from build123d import *

# Parameters (mm, degrees)
SKETCH1_W           = 100
SKETCH1_H           = 120
SKETCH1_R           = 2.6
SKETCH1_R_2         = 3.55
BOSS_EXTRUDE1_DEPTH = 3.2
FILLET1_R           = 10


with BuildPart() as part:
    # Sketch1 → Boss-Extrude1 (new body)
    with BuildSketch(Plane.XY):
        Rectangle(SKETCH1_W, SKETCH1_H)
        Circle(SKETCH1_R, mode=Mode.SUBTRACT)
        with Locations((0, 10)):
            Circle(SKETCH1_R, mode=Mode.SUBTRACT)
        with Locations((0, 42.3)):
            Circle(SKETCH1_R, mode=Mode.SUBTRACT)
        with Locations((0, -10)):
            Circle(SKETCH1_R, mode=Mode.SUBTRACT)
        with Locations((10, -20)):
            Circle(SKETCH1_R, mode=Mode.SUBTRACT)
        with Locations((10, 0)):
            Circle(SKETCH1_R, mode=Mode.SUBTRACT)
        with Locations((-10, 0)):
            Circle(SKETCH1_R, mode=Mode.SUBTRACT)
        with Locations((-32.3, 0)):
            Circle(SKETCH1_R_2, mode=Mode.SUBTRACT)
        with Locations((35.25, 0)):
            Circle(SKETCH1_R, mode=Mode.SUBTRACT)
        with Locations((35.25, 42.3)):
            Circle(SKETCH1_R, mode=Mode.SUBTRACT)
        with Locations((10, -30)):
            Circle(SKETCH1_R, mode=Mode.SUBTRACT)
        with Locations((-10, -20)):
            Circle(SKETCH1_R, mode=Mode.SUBTRACT)
        with Locations((-32.3, 42.3)):
            Circle(SKETCH1_R_2, mode=Mode.SUBTRACT)
        with Locations((-22.3, 42.3)):
            Circle(SKETCH1_R_2, mode=Mode.SUBTRACT)
        with Locations((-10, -30)):
            Circle(SKETCH1_R, mode=Mode.SUBTRACT)
        with Locations((-40, 10)):
            Circle(SKETCH1_R, mode=Mode.SUBTRACT)
        with Locations((-20, 10)):
            Circle(SKETCH1_R, mode=Mode.SUBTRACT)
        with Locations((20, 10)):
            Circle(SKETCH1_R, mode=Mode.SUBTRACT)
        with Locations((40, 10)):
            Circle(SKETCH1_R, mode=Mode.SUBTRACT)
        with Locations((40, -10)):
            Circle(SKETCH1_R, mode=Mode.SUBTRACT)
        with Locations((20, -10)):
            Circle(SKETCH1_R, mode=Mode.SUBTRACT)
        with Locations((-20, -10)):
            Circle(SKETCH1_R, mode=Mode.SUBTRACT)
        with Locations((-40, -10)):
            Circle(SKETCH1_R, mode=Mode.SUBTRACT)
        with Locations((25.25, 42.3)):
            Circle(SKETCH1_R, mode=Mode.SUBTRACT)
        with Locations((10, 42.3)):
            Circle(SKETCH1_R, mode=Mode.SUBTRACT)
        with Locations((-10, 42.3)):
            Circle(SKETCH1_R, mode=Mode.SUBTRACT)
        with Locations((-10, 30)):
            Circle(SKETCH1_R, mode=Mode.SUBTRACT)
        with Locations((-10, 20)):
            Circle(SKETCH1_R, mode=Mode.SUBTRACT)
        with Locations((10, 30)):
            Circle(SKETCH1_R, mode=Mode.SUBTRACT)
        with Locations((10, 20)):
            Circle(SKETCH1_R, mode=Mode.SUBTRACT)
        with Locations((-10, -42.3)):
            Circle(SKETCH1_R, mode=Mode.SUBTRACT)
        with Locations((10, -42.3)):
            Circle(SKETCH1_R, mode=Mode.SUBTRACT)
        with Locations((25.25, -42.3)):
            Circle(SKETCH1_R, mode=Mode.SUBTRACT)
        with Locations((-22.3, -42.3)):
            Circle(SKETCH1_R_2, mode=Mode.SUBTRACT)
        with Locations((-32.3, -42.3)):
            Circle(SKETCH1_R_2, mode=Mode.SUBTRACT)
        with Locations((35.25, -42.3)):
            Circle(SKETCH1_R, mode=Mode.SUBTRACT)
        with Locations((0, -42.3)):
            Circle(SKETCH1_R, mode=Mode.SUBTRACT)
    extrude(amount=BOSS_EXTRUDE1_DEPTH)

    # Fillet1
    fillet1_edges = [part.edges().sort_by_distance(p)[0] for p in [
        (50, -60, 1.6),
        (-50, -60, 1.6),
        (-50, 60, 1.6),
        (50, 60, 1.6),
    ]]
    fillet(fillet1_edges, radius=FILLET1_R)


solid = part.part
Part model, mm, in its own coordinate system. Coordinates: 2 decimals unless noted, no trailing zeros. Loops run counter-clockwise (first coordinate to the right, second up) from the corner with the lowest first, then second, coordinate; pieces in that order, holes last. Notation, with made-up numbers: (-32, -5.75) -> (18, -5.75) arc R26 ccw to (18, 17.25) -> close; hole circle Ø6 at (-11, -29). An arc over 180 degrees is marked (long way). Use a Markdown table: item, result. Add a question column.
Item 1: Band-saw the part on B-B on y = -30. Write the cut outline in (x, z), plus the area to 3 significant figures.
Item 2: Band-saw the part on A-A on x = -10. Give the number of separate pieces and of enclosed holes in the cut face, plus the area to 3 significant figures.
Item 3: Flat gauge pins, fed straight in: P1, Ø4, axis at x = -10, y = 30, coming from the +Z side; P2, Ø8.5, axis at x = 0, y = 0, coming from the -Z side. Where does each tip first touch, or does it go through?
Item 4: Pull direction Y, two halves, no side cores. Call faces 1 (the flat face through (50, -1, 2)), 2 (the cylindrical face through (-42.063, 8.418, 1.578)), 3 (the cylindrical face through (11.4, 32.19, 1.58)), 4 (the cylindrical face through (-47.15, -56.99, 1.62)): +Y half, -Y half, draft (parallel to the pull), parting line (faces both ways), or undercut.
Item 5: Band-saw the part on C-C on x = -24.5. Write the cut outline in (y, z).
Item 6: Probe probe 1 along Y at (x, z) = (-32.3, 1.7); probe 2 along Y at (x, z) = (35.25, 1.5); probe 3 along Y at (x, z) = (0, 2.45). List the from-to ranges inside material, lowest first.
Geometry says:
| question | item | result |
|---|---|---|
| 1 | outline | (-50, 0) -> (-12.6, 0) -> (-12.6, 3.2) -> (-50, 3.2) -> close; (-7.4, 0) -> (7.4, 0) -> (7.4, 3.2) -> (-7.4, 3.2) -> close; (12.6, 0) -> (50, 0) -> (50, 3.2) -> (12.6, 3.2) -> close |
| 1 | area | 287 mm² |
| 2 | separate pieces | 8 |
| 2 | enclosed holes | 0 |
| 2 | area | 268 mm² |
| 3 | P1 | through |
| 3 | P2 | z = 0 |
| 4 | face 1 | draft |
| 4 | face 2 | undercut |
| 4 | face 3 | undercut |
| 4 | face 4 | -Y half |
| 5 | outline | (-60, 0) -> (-45.09, 0) -> (-45.09, 3.2) -> (-60, 3.2) -> close; (-39.51, 0) -> (39.51, 0) -> (39.51, 3.2) -> (-39.51, 3.2) -> close; (45.09, 0) -> (60, 0) -> (60, 3.2) -> (45.09, 3.2) -> close |
| 6 | probe 1 | -60 to -45.85, -38.75 to -3.55, 3.55 to 38.75, 45.85 to 60 |
| 6 | probe 2 | -60 to -44.9, -39.7 to -2.6, 2.6 to 39.7, 44.9 to 60 |
| 6 | probe 3 | -60 to -44.9, -39.7 to -12.6, -7.4 to -2.6, 2.6 to 7.4, 12.6 to 39.7, 44.9 to 60 |
